```python
from build123d import *
from build123d.topology import SkipClean

# Parameters (mm, degrees)
SKETCH1_R               = 38.1
BOSS_EXTRUDE1_DEPTH     = 76.2
SHELL2_T                = 3.175
BOSS_EXTRUDE2_DEPTH     = 7
CUT_EXTRUDE1_DEPTH      = 99.527366122
CUT_EXTRUDE1_DEPTH_BACK = 99.527366122
SKETCH3_R               = 61.906276858
SKETCH3_R_2             = 41.275
SKETCH4_R               = 20.64
CUT_EXTRUDE2_DEPTH      = 7
SCALE1_SCALE            = 0.615384615


with BuildPart() as part:
    # Sketch1 → Boss-Extrude1 (new body)
    with BuildSketch(Plane(origin=(0, 0, 0), x_dir=(1, 0, 0), z_dir=(0, 1, 0))):
        with Locations(Location((0, 0, 0), (0, 0, 90))):
            Circle(SKETCH1_R)
    extrude(amount=BOSS_EXTRUDE1_DEPTH)

    # Shell2
    shell2_openings = [part.faces().sort_by_distance(p)[0] for p in [
        (0, 76.2, 0),
    ]]
    offset(amount=SHELL2_T, openings=shell2_openings, kind=Kind.INTERSECTION)

    # Sketch2 → Boss-Extrude2 (add)
    with BuildSketch(Plane(origin=(0, -3.175, 0), x_dir=(-1, 0, 0), z_dir=(0, -1, 0))):
        Polygon((-4.854101966, 0), (-39.718383202, -11.328091668), (-38.791332219, -14.181261217), (-3.927050983, -2.853169549), (-25.47436178, -32.510498564), (-23.047310797, -34.273854321), (-1.5, -4.616525306), (-1.5, -41.275), (1.5, -41.275), (1.5, -4.616525306), (23.047310797, -34.273854321), (25.47436178, -32.510498564), (3.927050983, -2.853169549), (38.791332219, -14.181261217), (39.718383202, -11.328091668), (4.854101966, 0), (39.718383202, 11.328091668), (38.791332219, 14.181261217), (3.927050983, 2.853169549), (25.47436178, 32.510498564), (23.047310797, 34.273854321), (1.5, 4.616525306), (1.5, 41.275), (-1.5, 41.275), (-1.5, 4.616525306), (-23.047310797, 34.273854321), (-25.47436178, 32.510498564), (-3.927050983, 2.853169549), (-38.791332219, 14.181261217), (-39.718383202, 11.328091668), align=None)
    extrude(amount=BOSS_EXTRUDE2_DEPTH)

    # Sketch3 → Cut-Extrude1 (cut, two sides: drawn at the far end of the back side and taken through both)
    with SkipClean():  # the faces are left unmerged after this step: merging them gives an invalid solid
        with BuildSketch(Plane.XZ.offset(3.175).offset(-CUT_EXTRUDE1_DEPTH_BACK)):
            Circle(SKETCH3_R)
            with Locations(Location((0, 0, 0), (0, 0, 272.082679548))):
                Circle(SKETCH3_R_2, mode=Mode.SUBTRACT)
        extrude(amount=CUT_EXTRUDE1_DEPTH + CUT_EXTRUDE1_DEPTH_BACK, mode=Mode.SUBTRACT)

    # Sketch4 → Cut-Extrude2 (cut)
    with SkipClean():  # the faces are left unmerged after this step: merging them gives an invalid solid
        with BuildSketch(Plane.XZ.offset(10.175)):
            Circle(SKETCH4_R)
        extrude(amount=-CUT_EXTRUDE2_DEPTH, mode=Mode.SUBTRACT)


with BuildPart() as part_1:
    # Scale1: scaled about (0, 27.463968189, 0)
    add(part.part.scale(SCALE1_SCALE).moved(Location((0, 10.563064688, 0))))


solid = part_1.part
```
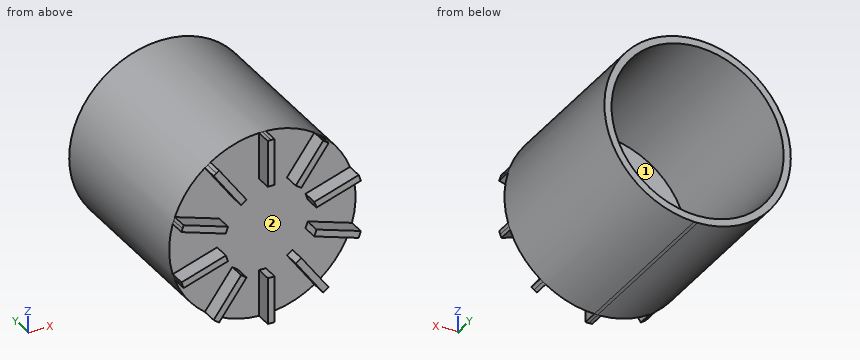
Here's how the part is built. I have some questions about the finished solid (model axes, mm). Face numbers are marked on the shaded views. Coordinates: 2 decimals unless noted, no trailing zeros. Order: outer loops, then holes, each group sorted by start corner. A loop starts at its lowest first (then second) coordinate and runs counter-clockwise, first axis right, second up. Notation, with made-up numbers: (-40, 2) - (17, 2) arc R19 cw to (17, 36) - close; hole circle Ø7 at (13.5, 47). An arc over 180 degrees is marked (long way). One line per question, with ' | ' between items.
(1) Suppose I cut it at D-D on z = 17. List the corners of the cut face in (x, y) for me.
Report:
outline: (-18.87, 8.61) - (-13.49, 8.61) - (-13.49, 4.3) - (-11.21, 4.3) - (-11.21, 8.61) - (-0.92, 8.61) - (-0.92, 4.3) - (0.92, 4.3) - (0.92, 8.61) - (11.21, 8.61) - (11.21, 4.3) - (13.49, 4.3) - (13.49, 8.61) - (18.87, 8.61) - (18.87, 57.46) - (16.15, 57.46) - (16.15, 10.56) - (-16.15, 10.56) - (-16.15, 57.46) - (-18.87, 57.46) - close
(2) If we mould it in two halves opening along X, with no side actions, what happens to the marked faces 1 and 2? For each: pulls with the +X half, pulls with the -X half, needs draft (parallel to the pull), parting line crosses it, or undercut.
Report:
face 1: undercut | face 2: undercut
(3) Suppose I cut it at C-C on y = 21. List the corners of the cut face in (x, z) for me, and give its area (3 significant figures).
Report:
outline: circle Ø50.8 at (0, 0); hole circle Ø46.89 at (0, 0) | area: 300 mm2
(4) Will these pins go through, and if not, where does the flat tip stop? pin 1 (1 mm diameter, centred on x = -8, y = 25.5, fed in from -Z); pin 2 (1 mm diameter, centred on x = -15, y = 51.5, fed in from +Z); pin 3 (2 mm diameter, centred on y = 6, z = 19.5, fed in from -X).
Report:
pin 1: stops at z = -24.27 | pin 2: stops at z = 20.85 | pin 3: stops at x = -15.67
(5) Suppose I cut it at A-A on z = 0. List the corners of the cut face in (x, y) for me, and give its area (3 significant figures).
Report:
outline: (-25.4, 8.61) - (25.4, 8.61) - (25.4, 57.46) - (23.45, 57.46) - (23.45, 10.56) - (-23.45, 10.56) - (-23.45, 57.46) - (-25.4, 57.46) - close | area: 282 mm2
(6) Suppose I cut it at B-B on x = 19.5. List the corners of the cut face in (y, z) for me, and give its area (3 significant figures).
Report:
outline: (4.3, -7.31) - (8.61, -7.31) - (8.61, -16.28) - (57.46, -16.28) - (57.46, -13.02) - (10.56, -13.02) - (10.56, 13.02) - (57.46, 13.02) - (57.46, 16.28) - (8.61, 16.28) - (8.61, 7.31) - (4.3, 7.31) - (4.3, 5.37) - (8.61, 5.37) - (8.61, -5.37) - (4.3, -5.37) - close | area: 386 mm2
(7) If I drill on L1, parallel to X at y = 40, z = 0; L2, parallel to Z at x = -8.5, y = 51; L3, parallel to Y at x = -10, z = -6.5, over which ranges is the centre line in solid material (lowest first)?
Report:
L1: x = -25.4 to -23.45, 23.45 to 25.4 | L2: z = -23.94 to -21.85, 21.85 to 23.94 | L3: y = 8.61 to 10.56
